```python
from build123d import *

# Parameters (mm, degrees)
CROQUIS1_W              = 560
CROQUIS1_H              = 1200
CROQUIS1_W_2            = 530
CROQUIS1_H_2            = 1170
SALIENTE_EXTRUIR1_DEPTH = 15
REDONDEO1_R             = 2
REDONDEO2_R             = 2
CROQUIS2_R              = 3.75
SALIENTE_EXTRUIR2_DEPTH = 15
CROQUIS3_R              = 5
CORTAR_EXTRUIR1_DEPTH   = 576
ESCALA1_SCALE           = 1.3


with BuildPart() as part:
    # Croquis1 → Saliente-Extruir1 (new body)
    with BuildSketch(Plane(origin=(0, 0, 0), x_dir=(1, 0, 0), z_dir=(0, 1, 0))):
        Rectangle(CROQUIS1_W, CROQUIS1_H)
        Rectangle(CROQUIS1_W_2, CROQUIS1_H_2, mode=Mode.SUBTRACT)
    extrude(amount=SALIENTE_EXTRUIR1_DEPTH)

    # Redondeo1
    redondeo1_edges = [part.edges().sort_by_distance(p)[0] for p in [
        (-280, 15, 0),
        (265, 15, 0),
        (0, 15, 600),
        (0, 15, -585),
        (-265, 15, 0),
        (0, 15, 585),
        (280, 15, 0),
        (0, 15, -600),
    ]]
    fillet(redondeo1_edges, radius=REDONDEO1_R)

    # Redondeo2
    redondeo2_edges = [part.edges().sort_by_distance(p)[0] for p in [
        (265, 0, 0),
        (0, 0, -585),
        (-265, 0, 0),
        (0, 0, 585),
        (0, 0, 600),
        (-280, 0, 0),
        (0, 0, -600),
        (280, 0, 0),
    ]]
    fillet(redondeo2_edges, radius=REDONDEO2_R)

    # Croquis2 → Saliente-Extruir2 (add)
    with BuildSketch(Plane.ZY.offset(280)):
        with Locations((596.25, 7.5)):
            Circle(CROQUIS2_R)
        with Locations((-596.25, 7.5)):
            Circle(CROQUIS2_R)
    saliente_extruir2 = extrude(amount=SALIENTE_EXTRUIR2_DEPTH)

    # Simetría1: Saliente-Extruir2 across plane
    add(saliente_extruir2.mirror(Plane(origin=(0, 0, 0), x_dir=(0, 0, 1), z_dir=(1, 0, 0))))

    # Croquis3 → Cortar-Extruir1 (cut, through all)
    with BuildSketch(Plane.ZY.offset(280)):
        with Locations((0, 7.5)):
            Circle(CROQUIS3_R)
    extrude(amount=-CORTAR_EXTRUIR1_DEPTH, mode=Mode.SUBTRACT)


with BuildPart() as part_1:
    # Escala1: scaled about (0, 0, 0)
    add(part.part.scale(ESCALA1_SCALE))


solid = part_1.part
```
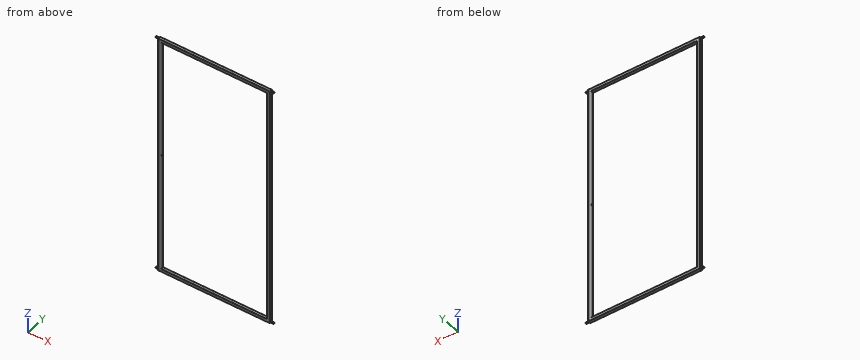
Geometry: final body of the model. Coordinates: model frame, mm. Round coordinates to 2 decimals unless told otherwise and drop trailing zeros. Write each loop counter-clockwise with the first axis right and the second up, starting at its lowest first coordinate (ties: lowest second). Pieces come first, ordered by that corner, then holes. Notation, with made-up numbers: (81, -14.75) -> (136, -14.75) arc R35 cw to (136, 24.25) -> close; hole circle Ø10 at (53, -3). An arc over 180 degrees is marked (long way). Return JSON: item names as keys, results as strings.
Q1. Section A-A on z = 34. Return the cut outline in (x, y).
From the geometry:
{"outline": "(-364, 2.6) arc R2.6 ccw to (-361.4, 0) -> (-347.1, 0) arc R2.6 ccw to (-344.5, 2.6) -> (-344.5, 16.9) arc R2.6 ccw to (-347.1, 19.5) -> (-361.4, 19.5) arc R2.6 ccw to (-364, 16.9) -> close; (344.5, 2.6) arc R2.6 ccw to (347.1, 0) -> (361.4, 0) arc R2.6 ccw to (364, 2.6) -> (364, 16.9) arc R2.6 ccw to (361.4, 19.5) -> (347.1, 19.5) arc R2.6 ccw to (344.5, 16.9) -> close"}
Q2. Section B-B on x = -175. Return the cut outline in (y, z).
From the geometry:
{"outline": "(0, -777.4) arc R2.6 ccw to (2.6, -780) -> (16.9, -780) arc R2.6 ccw to (19.5, -777.4) -> (19.5, -763.1) arc R2.6 ccw to (16.9, -760.5) -> (2.6, -760.5) arc R2.6 ccw to (0, -763.1) -> close; (0, 763.1) arc R2.6 ccw to (2.6, 760.5) -> (16.9, 760.5) arc R2.6 ccw to (19.5, 763.1) -> (19.5, 777.4) arc R2.6 ccw to (16.9, 780) -> (2.6, 780) arc R2.6 ccw to (0, 777.4) -> close"}
Q3. Ray query, line 1 (X direction, y = 13.5, z = 213.5); line 2 (Z direction, x = -293, y = 7); line 3 (Y direction, x = -352.25, z = 0). Return the intervals inside material, ascending.
From the geometry:
{"line 1": "-364 to -344.5, 344.5 to 364", "line 2": "-780 to -760.5, 760.5 to 780", "line 3": "0 to 3.25, 16.25 to 19.5"}
Q4. First-contact query: pin 1 Ø7 at (y, z) = (13, 247) entering from -X; pin 2 Ø7 at (y, z) = (11.5, -30) entering from +X; pin 3 Ø4.5 at (y, z) = (12, 0) entering from -X. Flat tips, straight axial feed; report the tip coordinate or a pass-through.
From the geometry:
{"pin 1": "x = -364", "pin 2": "x = 364", "pin 3": "through"}
